The listing builds one solid part. Answer for the finished solid, in the listing's coordinates (mm). A direction names the side the tool comes from. Round coordinates to 2 decimals unless told otherwise and drop trailing zeros. Write each loop counter-clockwise with the first axis right and the second up, starting at its lowest first coordinate (ties: lowest second). Pieces come first, ordered by that corner, then holes. Notation, with made-up numbers: (-38.75, 66) - (-9.75, 66) arc R25 cw to (-9.75, 93) - close; hole circle Ø9 at (-18.5, -3). An arc over 180 degrees is marked (long way). Answer as CSV lines item,"result". Start each with the question number.
Item 1: Straight lines are drawn through the part: line 1 along Z through (x, y) = (-5, 27.75); line 2 along Y through (x, z) = (37.5, 1.5); line 3 along X through (y, z) = (18.5, 12). For each, find the intervals that lie inside material, in ascending order. Write a range as [from, to].
Item 2: Flat-ended cylindrical pins translate along their axes: pin 1 (1 mm diameter, centred on y = 16, z = 12, fed in from -X); pin 2 (1.2 mm diameter, centred on x = 44, y = 27.5, fed in from +Z); pin 3 (5 mm diameter, centred on x = 45.5, z = 15, fed in from +Y). Find the tip coordinate at first contact, or state that the pin passes through.
Item 3: Which of the six approach directions +Z, -Z, +X, -X, +Y, -Y give full straight-line access (tool end or side, diameter ignored) to faces 4 (the flat face through (44, 28, 19)), 5 (the flat face through (42, 2, 13)), 6 (the flat face through (43, 26.6, 10))?
Item 4: A cutting plane is placed at D-D on y = 12. Determine the outline of the cut face in (x, z).
Item 5: A cutting plane is placed at A-A on x = -5. Determine the outline of the cut face in (y, z), and give its area (3 significant figures).
Item 6: A cutting plane is placed at B-B on z = 11.5. Determine the outline of the cut face in (x, y).
Item 7: A cutting plane is placed at C-C on x = 30.1. Determine the outline of the cut face in (y, z), and give its area (3 significant figures).
Item 8: For a pull along Y with two mould halves and no side action, classify faces 1 (the flat face through (40.5, 18, 10)), 2 (the flat face through (28, 36.1, 8)), 3 (the flat face through (47.5, 28, 10)) as pulls with the +Y half, pulls with the -Y half, needs draft (parallel to the pull), parting line crosses it, or undercut.
```python
from build123d import *

# Parameters (mm, degrees)
SKETCH1_W           = 40.5
SKETCH1_H           = 36.1
BOSS_EXTRUDE1_DEPTH = 20
BOSS_EXTRUDE2_START = -1
SKETCH2_W           = 7
SKETCH2_H           = 2.5
BOSS_EXTRUDE2_DEPTH = 18
CUT_EXTRUDE1_REACH  = 61.187
SKETCH4_R           = 2.5
BOSS_EXTRUDE3_DEPTH = 6
BOSS_EXTRUDE4_START = -7
BOSS_EXTRUDE4_DEPTH = 6
CUT_EXTRUDE2_REACH  = 68.548


with BuildPart() as part:
    # Sketch1 → Boss-Extrude1 (new body)
    with BuildSketch(Plane.XY):
        with Locations((20.25, 18.05)):
            Rectangle(SKETCH1_W, SKETCH1_H)
    extrude(amount=BOSS_EXTRUDE1_DEPTH)

    # Sketch2 → Boss-Extrude2 (add)
    with BuildSketch(Plane.XY.offset(20).offset(BOSS_EXTRUDE2_START)):
        with Locations((-3.5, 27.85)):
            Rectangle(SKETCH2_W, SKETCH2_H)
        with Locations((44, 27.85)):
            Rectangle(SKETCH2_W, SKETCH2_H)
    extrude(amount=-BOSS_EXTRUDE2_DEPTH)

    # Sketch3 → Cut-Extrude1 (cut, up to next)
    with BuildSketch(Plane(origin=(0, 29.1, 0), x_dir=(1, 0, 0), z_dir=(0, 1, 0)), mode=Mode.PRIVATE) as cut_extrude1_sk1:
        with BuildLine():
            Line((-6.870828693, -3.75), (-7, -3.75))
            Line((-7, -3.75), (-7, -6.25))
            Line((-7, -6.25), (-6.870828693, -6.25))
            ThreePointArc((-6.870828693, -6.25), (-2.75, -5), (-6.870828693, -3.75))
        make_face()
    cut_extrude1_tool1 = extrude(cut_extrude1_sk1.sketch, amount=-CUT_EXTRUDE1_REACH, mode=Mode.PRIVATE) & part.part
    # Sketch3 → Cut-Extrude1 (cut, up to next)
    with BuildSketch(Plane(origin=(0, 29.1, 0), x_dir=(1, 0, 0), z_dir=(0, 1, 0)), mode=Mode.PRIVATE) as cut_extrude1_sk2:
        with BuildLine():
            Line((-7, -13.75), (-6.870828693, -13.75))
            ThreePointArc((-6.870828693, -13.75), (-2.75, -15), (-6.870828693, -16.25))
            Line((-6.870828693, -16.25), (-7, -16.25))
            Line((-7, -16.25), (-7, -13.75))
        make_face()
    cut_extrude1_tool2 = extrude(cut_extrude1_sk2.sketch, amount=-CUT_EXTRUDE1_REACH, mode=Mode.PRIVATE) & part.part
    # Sketch3 → Cut-Extrude1 (cut, up to next)
    with BuildSketch(Plane(origin=(0, 29.1, 0), x_dir=(1, 0, 0), z_dir=(0, 1, 0)), mode=Mode.PRIVATE) as cut_extrude1_sk3:
        with BuildLine():
            Line((47.370828693, -16.25), (47.5, -16.25))
            Line((47.5, -16.25), (47.5, -13.75))
            Line((47.5, -13.75), (47.370828693, -13.75))
            ThreePointArc((47.370828693, -13.75), (43.25, -15), (47.370828693, -16.25))
        make_face()
    cut_extrude1_tool3 = extrude(cut_extrude1_sk3.sketch, amount=-CUT_EXTRUDE1_REACH, mode=Mode.PRIVATE) & part.part
    # Sketch3 → Cut-Extrude1 (cut, up to next)
    with BuildSketch(Plane(origin=(0, 29.1, 0), x_dir=(1, 0, 0), z_dir=(0, 1, 0)), mode=Mode.PRIVATE) as cut_extrude1_sk4:
        with BuildLine():
            Line((47.5, -6.25), (47.370828693, -6.25))
            ThreePointArc((47.370828693, -6.25), (43.25, -5), (47.370828693, -3.75))
            Line((47.370828693, -3.75), (47.5, -3.75))
            Line((47.5, -3.75), (47.5, -6.25))
        make_face()
    cut_extrude1_tool4 = extrude(cut_extrude1_sk4.sketch, amount=-CUT_EXTRUDE1_REACH, mode=Mode.PRIVATE) & part.part
    add(cut_extrude1_tool1.solids().sort_by_distance((-4.956552, 29.1, 5))[0], mode=Mode.SUBTRACT)
    add(cut_extrude1_tool2.solids().sort_by_distance((-4.956552, 29.1, 15))[0], mode=Mode.SUBTRACT)
    add(cut_extrude1_tool3.solids().sort_by_distance((45.456552, 29.1, 15))[0], mode=Mode.SUBTRACT)
    add(cut_extrude1_tool4.solids().sort_by_distance((45.456552, 29.1, 5))[0], mode=Mode.SUBTRACT)

    # Sketch4 → Boss-Extrude3 (add)
    with BuildSketch(Plane(origin=(0, 36.1, 0), x_dir=(1, 0, 0), z_dir=(0, 1, 0))):
        with Locations(Location((30.1, -10, 0), (0, 0, 90))):
            Circle(SKETCH4_R)
    extrude(amount=BOSS_EXTRUDE3_DEPTH)

    # Sketch5 → Boss-Extrude4 (add)
    with BuildSketch(Plane.XY.offset(20).offset(BOSS_EXTRUDE4_START)):
        Polygon((40.5, 4), (41.5, 4), (41.5, 3.5), (45.5, 2.794692077), (45.5, 1.794692077), (41.5, 1.089384154), (41.5, 0.589384154), (40.5, 0.589384154), align=None)
    extrude(amount=-BOSS_EXTRUDE4_DEPTH)

    # Sketch6 → Cut-Extrude2 (cut, up to next)
    with BuildSketch(Plane.XY.offset(20), mode=Mode.PRIVATE) as cut_extrude2_sk1:
        Polygon((0, 32.6), (19.849486369, 36.1), (0, 36.1), align=None)
    cut_extrude2_tool1 = extrude(cut_extrude2_sk1.sketch, amount=-CUT_EXTRUDE2_REACH, mode=Mode.PRIVATE) & part.part
    add(cut_extrude2_tool1.solids().sort_by_distance((6.616495, 34.933333, 20))[0], mode=Mode.SUBTRACT)


solid = part.part
```
Geometry says:
1,line 1,"z = [1, 2.75], [7.25, 12.75], [17.25, 19]"
1,line 2,"y = [0, 36.1]"
1,line 3,"x = [0, 40.5]"
2,pin 1,"stops at x = 0"
2,pin 2,"stops at z = 19"
2,pin 3,"stops at y = 29.1"
3,face 4,"+Z, +X, +Y, -Y"
3,face 5,"+Z, +X, -Y"
3,face 6,"+Z, -Z, +X"
4,outline,"(0, 0) - (40.5, 0) - (40.5, 20) - (0, 20) - close"
5,outline,"(26.6, 1) - (29.1, 1) - (29.1, 2.75) - (26.6, 2.75) - close; (26.6, 7.25) - (29.1, 7.25) - (29.1, 12.75) - (26.6, 12.75) - close; (26.6, 17.25) - (29.1, 17.25) - (29.1, 19) - (26.6, 19) - close"
5,area,"22.5 mm^2"
6,outline,"(-7, 26.6) - (0, 26.6) - (0, 0) - (40.5, 0) - (40.5, 0.59) - (41.5, 0.59) - (41.5, 1.09) - (45.5, 1.79) - (45.5, 2.79) - (41.5, 3.5) - (41.5, 4) - (40.5, 4) - (40.5, 26.6) - (47.5, 26.6) - (47.5, 29.1) - (40.5, 29.1) - (40.5, 36.1) - (32.1, 36.1) - (32.1, 42.1) - (28.1, 42.1) - (28.1, 36.1) - (19.85, 36.1) - (0, 32.6) - (0, 29.1) - (-7, 29.1) - close"
7,outline,"(0, 0) - (36.1, 0) - (36.1, 7.5) - (42.1, 7.5) - (42.1, 12.5) - (36.1, 12.5) - (36.1, 20) - (0, 20) - close"
7,area,"752 mm^2"
8,face 1,"undercut"
8,face 2,"pulls with the +Y half"
8,face 3,"needs draft"
